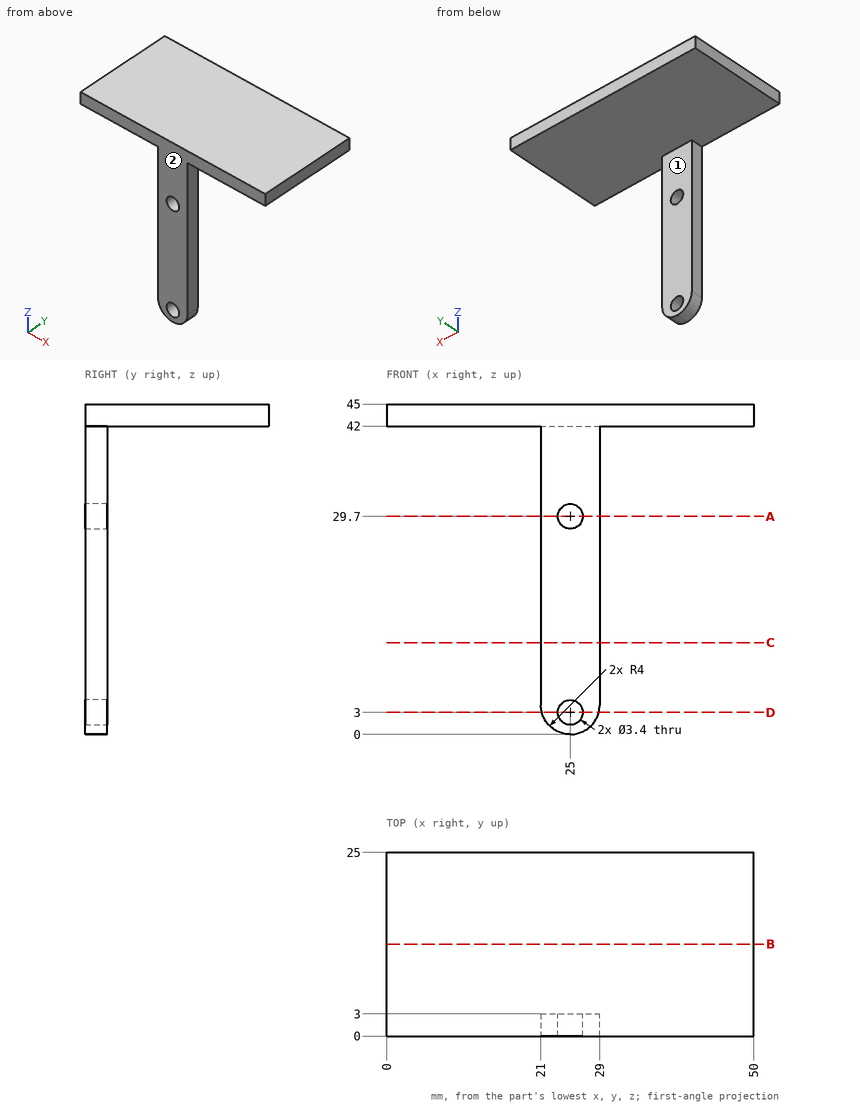
Can you work these out from the drawing? Everything is in mm from the part's minimum corner. A direction names the side the tool comes from. Round coordinates to 2 decimals unless told otherwise and drop trailing zeros. Loops run counter-clockwise (first coordinate to the right, second up) from the corner with the lowest first, then second, coordinate; pieces in that order, holes last. Notation, with made-up numbers: (68.5, 58.5) -> (122.5, 58.5) arc R28 ccw to (122.5, 93.5) -> close; hole circle Ø3 at (14.5, -21.5). An arc over 180 degrees is marked (long way). Use CSV: the item, a comma, the result in double quotes.
(1) If I drill on probe 1 along X at (y, z) = (1.45, 29.7); probe 2 along X at (y, z) = (1.75, 5.5); probe 3 along Z at (x, y) = (19.5, 12.5), over which ranges is the centre line in solid material (lowest first)? Write a range as [from, to].
Return value:
probe 1,"x = [21, 23.3], [26.7, 29]"
probe 2,"x = [21, 29]"
probe 3,"z = [42, 45]"
(2) Will these pins go through, and if not, where does the flat tip stop? pin 1 Ø10 at (x, z) = (18.5, 16) entering from +Y; pin 2 Ø3.5 at (y, z) = (1.5, 16.5) entering from -X; pin 3 Ø2 at (x, z) = (25, 29.7) entering from -Y; pin 4 Ø1 at (x, y) = (38.5, 11) entering from -Z.
Return value:
pin 1,"stops at y = 3"
pin 2,"stops at x = 21"
pin 3,"passes through"
pin 4,"stops at z = 42"
(3) For the marked faces 1 and 2, which set-ups out of +Z, -Z, +X, -X, +Y, -Y let a thin tool reach every point of the face, with its end or its side?
Return value:
face 1,"-Z, +X, -X, +Y"
face 2,"+Z, -Z, +X, -X, -Y"
(4) Suppose I cut it at B-B on y = 12.5. Write out the boundary of the cut face in (x, z).
Return value:
outline,"(0, 42) -> (50, 42) -> (50, 45) -> (0, 45) -> close"
(5) Suppose I cut it at A-A on z = 29.7. Write out the boundary of the cut face in (x, y), plus the area to 3 significant figures.
Return value:
outline,"(21, 0) -> (23.3, 0) -> (23.3, 3) -> (21, 3) -> close; (26.7, 0) -> (29, 0) -> (29, 3) -> (26.7, 3) -> close"
area,"13.8 mm²"
(6) Suppose I cut it at C-C on z = 12.5. Write out the boundary of the cut face in (x, y), plus the area to 3 significant figures.
Return value:
outline,"(21, 0) -> (29, 0) -> (29, 3) -> (21, 3) -> close"
area,"24.0 mm²"
(7) Suppose I cut it at D-D on z = 3. Write out the boundary of the cut face in (x, y), plus the area to 3 significant figures.
Return value:
outline,"(21.13, 0) -> (23.3, 0) -> (23.3, 3) -> (21.13, 3) -> close; (26.7, 0) -> (28.87, 0) -> (28.87, 3) -> (26.7, 3) -> close"
area,"13.0 mm²"
